Design review of the part built by this model. Coordinates are the model's own, in mm. Face numbers are marked on the shaded views. Coordinates: 2 decimals unless noted, no trailing zeros. Loops run counter-clockwise (first coordinate to the right, second up) from the corner with the lowest first, then second, coordinate; pieces in that order, holes last. Notation, with made-up numbers: M 59.25,-3.5 L 104.25,-3.5 A23 cw 104.25,8.5 Z; hole C 81,13 d10. An arc over 180 degrees is marked long. Put each result on its own line as item: value. Start each with the question number.
(1) The part is to be moulded in two halves that separate along X. For the marked faces 1, 2 and 3, say which applies: +X half, -X half, draft (parallel to the pull), parting line (faces both ways), or undercut.
(2) Clearance check with flat-ended pins moving along their axes: pin 1 (1 mm diameter, centred on x = -3.6, z = 5.08, fed in from +Y); pin 2 (3 mm diameter, centred on x = 6, z = 67, fed in from +Y); pin 3 (3 mm diameter, centred on x = -1, z = 88.5, fed in from +Y); pin 4 (1.5 mm diameter, centred on y = 1.5, z = 24.5, fed in from +X). State where each tip first meets the part, or that it passes through.
(3) For probe 1 along X at (y, z) = (6.25, 5.08); probe 2 along Y at (x, z) = (-21, 38); probe 3 along X at (y, z) = (4, 89), list the stretches that pass through material, from the lowest coordinate up. Write a range as [from, to].
(4) Take a section at A-A, the plane z = 82.5. Give the boundary of the cut face in (x, y).
(5) Take a section at B-B, the plane x = -10. Give the boundary of the cut face in (y, z).
```python
from build123d import *

# Parameters (mm, degrees)
BOSS_EXTRUDE1_DEPTH                = 127
SKETCH4_R                          = 1.27
BOSS_EXTRUDE2_DEPTH                = 5.08
F_1_16_0_0625_DIAMETER_HOLE1_D     = 1.5875
F_1_16_0_0625_DIAMETER_HOLE1_DEPTH = 7.478589674


with BuildPart() as part:
    # Sketch1 → Boss-Extrude1 (new body)
    with BuildSketch(Plane.XY):
        with BuildLine():
            Line((-33.131044693, 0), (2.017058644, 0))
            ThreePointArc((2.017058644, 0), (5.688774014, 1.520874304), (7.209648317, 5.192589674))
            Line((7.209648317, 5.192589674), (4.272091587, 5.192589674))
            ThreePointArc((4.272091587, 5.192589674), (3.453747934, 3.216933327), (1.478091587, 2.398589674))
            Line((1.478091587, 2.398589674), (-32.989634367, 2.398589674))
            ThreePointArc((-32.989634367, 2.398589674), (-34.965290713, 3.216933327), (-35.783634367, 5.192589674))
            Line((-35.783634367, 5.192589674), (-38.323634367, 5.192589674))
            ThreePointArc((-38.323634367, 5.192589674), (-36.802760063, 1.520874304), (-33.131044693, 0))
        make_face()
    extrude(amount=BOSS_EXTRUDE1_DEPTH)

    # Sketch4 → Boss-Extrude2 (add)
    with BuildSketch(Plane(origin=(0, 2.398589674, 0), x_dir=(1, 0, 0), z_dir=(0, 1, 0))):
        with Locations((-27.909634367, -5.08)):
            Circle(SKETCH4_R)
        with Locations((-3.601908413, -5.08)):
            Circle(SKETCH4_R)
        with Locations((-27.909634367, -121.964874012)):
            Circle(SKETCH4_R)
        with Locations((-3.601908413, -121.964874012)):
            Circle(SKETCH4_R)
    extrude(amount=BOSS_EXTRUDE2_DEPTH)

    # 1/16 (0.0625) Diameter Hole1
    with Locations(Plane(origin=(0, 7.478589674, 0), x_dir=(1, 0, 0), z_dir=(0, 1, 0))):
        with Locations((-27.909634367, -5.08), (-3.601908413, -5.08), (-27.909634367, -121.964874012), (-3.601908413, -121.964874012)):
            Hole(F_1_16_0_0625_DIAMETER_HOLE1_D / 2, depth=F_1_16_0_0625_DIAMETER_HOLE1_DEPTH)


solid = part.part
```
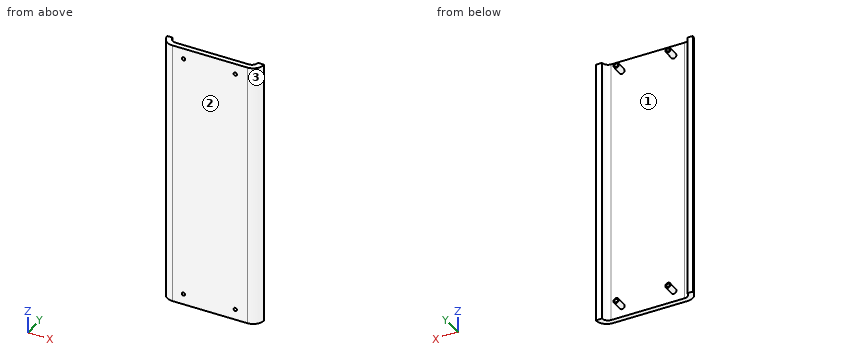
Computed values:
1. face 1: undercut
1. face 2: draft
1. face 3: +X half
2. pin 1: passes through
2. pin 2: stops at y = 5.19
2. pin 3: stops at y = 2.4
2. pin 4: stops at x = 6.3
3. probe 1: x = [-29.18, -28.7], [-27.12, -26.64], [-4.87, -4.4], [-2.81, -2.33]
3. probe 2: y = [0, 2.4]
3. probe 3: x = [-38.18, -35.52], [4, 7.07]
4. outline: M -38.32,5.19 A5.19 ccw -33.13,0 L 2.02,0 A5.19 ccw 7.21,5.19 L 4.27,5.19 A2.79 cw 1.48,2.4 L -32.99,2.4 A2.79 cw -35.78,5.19 Z
5. outline: M 0,0 L 2.4,0 L 2.4,127 L 0,127 Z
